Read the model definition and answer for the solid it produces. Units are mm, in the model's axes. Face numbers are marked on the shaded views. A direction names the side the tool comes from. Round coordinates to 2 decimals unless told otherwise and drop trailing zeros. Order: outer loops, then holes, each group sorted by start corner. A loop starts at its lowest first (then second) coordinate and runs counter-clockwise, first axis right, second up. Notation, with made-up numbers: (40.25, 29) - (64.25, 29) arc R27 cw to (64.25, 60) - close; hole circle Ø10 at (50, -19.75). An arc over 180 degrees is marked (long way). Put each result on its own line as item: value. Start each with the question number.
Q1. Which of the six approach directions +Z, -Z, +X, -X, +Y, -Y give full straight-line access (tool end or side, diameter ignored) to the marked faces 4 and 5?
Q2. Find the intervals of material crossed by line 1 along X through (y, z) = (10.5, 21); line 2 along Y through (x, z) = (29, 48.5); line 3 along X through (y, z) = (22.5, 43), in increasing order. Write a range as from..to.
Q3. For a pull along X with two mould halves and no side action, classify the marked faces 1, 2 and 3 as pulls with the +X half, pulls with the -X half, needs draft (parallel to the pull), parting line crosses it, or undercut.
Q4. Section C-C on y = 7.75 is taken. Give the vertices of the cut face in (x, z).
Q5. Section B-B on z = 31 is taken. Give the vertices of the cut face in (x, y).
Q6. Section D-D on x = 9.5 is taken. Give the vertices of the cut face in (y, z).
Q7. Each of these flat-tipped pins is pushed along its axis until it touches: pin 1 Ø8 at (x, y) = (16.5, 20.5) entering from +Z; pin 2 Ø22.5 at (x, z) = (25, 67.5) entering from +Y; pin 3 Ø2.5 at (x, y) = (7.5, 18.5) entering from -Z. Where does it stop, or does it pass through?
Q8. Section A-A on y = 21.5 is taken. Give the vertices of the cut face in (x, z), then the cut area to 3 significant figures.
Autodesk Inventor part; units mm, degrees
ref_plane "YZ Plane" through (0, 0, 0) normal (1, 0, 0) x (0, 1, 0)
ref_plane "XZ Plane" through (0, 0, 0) normal (0, 1, 0) x (-1, 0, 0)
ref_plane "XY Plane" through (0, 0, 0) normal (0, 0, 1) x (1, 0, 0)
sketch "Sketch1" plane through (0, 0, 0) normal (0, 0, 1) x (1, 0, 0)
  line L0 (10.7104, 9.7791) -> (45.7104, 9.7791)
  line L1 (45.7104, 9.7791) -> (45.7104, 24.7791)
  line L2 (10.7104, 9.7791) -> (10.7104, 24.7791)
  line L3 (5.7104, 24.7791) -> (5.7104, 4.7791)
  line L4 (5.7104, 4.7791) -> (50.7104, 4.7791)
  line L5 (50.7104, 4.7791) -> (50.7104, 24.7791)
  line L6 (5.7104, 24.7791) -> (10.7104, 24.7791)
  line L7 (45.7104, 24.7791) -> (50.7104, 24.7791)
  point P0 (0, 0)
  point P1 (28.2104, 9.7791)
  dimension "d0" = 35
  dimension "d1" = 15
  dimension "d2" = 15
  dimension "d29" = 5
extrude "Extrusion1" add sketch "Sketch1" along normal blind 100
sketch "Sketch3" plane through (10.7104, 9.7791, 0) normal (0, 1, 0) x (1, 0, 0)
  line L0 (-5, -100) -> (40, -100)
  line L1 (-5, 0) -> (-5, -100)
  line L2 (17.5, -100) -> (37.1919, -100) construction
  line L3 (-5, -85.7353) -> (-5, -100)
  line L4 (-5, -100) -> (17.5, -100)
  line L5 (40, 0) -> (40, -100)
  line L6 (17.5, -100) -> (37.1919, -100) construction
  line L7 (40, -85.7353) -> (40, -100)
  line L8 (40, -100) -> (17.5, -100)
  line L9 (40, 0) -> (40, -100)
  line L10 (17.5, -100) -> (-5, -36.462)
  line L11 (17.5, -100) -> (40, -36.462)
  line L12 (-5, -36.462) -> (40, -36.462)
  line L13 (35, 0) -> (35, -100)
  line L14 (0, 0) -> (0, -100)
  point P0 (-10.7104, 0)
  point P1 (-5, -77.7514)
  point P2 (40, -36.462)
  point P3 (-5, -60.8533)
  dimension "d33" = 39
extrude "Extrusion5" cut sketch "Sketch3" along normal through all both and the other way through all contours L1 L10 L14 L0 | L14 L10 L0 | L11 L13 L0 | L13 L11 L5 L0
sketch "Sketch4" plane through (50.7104, 4.7791, 0) normal (1, 0, 0) x (0, 0, -1)
  line L0 (0, 20) -> (-50.5815, 20)
  line L1 (0, 20) -> (-4, 20)
  line L2 (-4, 20) -> (-4, 5)
  line L3 (0, 5) -> (-50.5815, 5)
  line L4 (0, 20) -> (0, 5)
  line L5 (0, 5) -> (0, 20)
  line L6 (0, 20) -> (0, 5)
  line L7 (-4, 5) -> (0, 5)
  point P0 (0, -4.7791)
  dimension "d24" = 4
extrude "Extrusion6" cut sketch "Sketch4" against normal through all
equation "\"BendRadius\" = Thickness"
equation "\"BendReliefWidth\" = Thickness"
equation "\"BendReliefDepth\" = 0.5 * Thickness"
equation "\"CornerReliefSize\" = 4 * Thickness"
equation "\"MinimumRemnant\" = 2 * Thickness"
equation "\"TransitionRadius\" = BendRadius"
equation "\"JacobiRadiusSize\" = BendRadius"
equation "\"GapSize\" = Thickness"
properties part number "middleslide2"
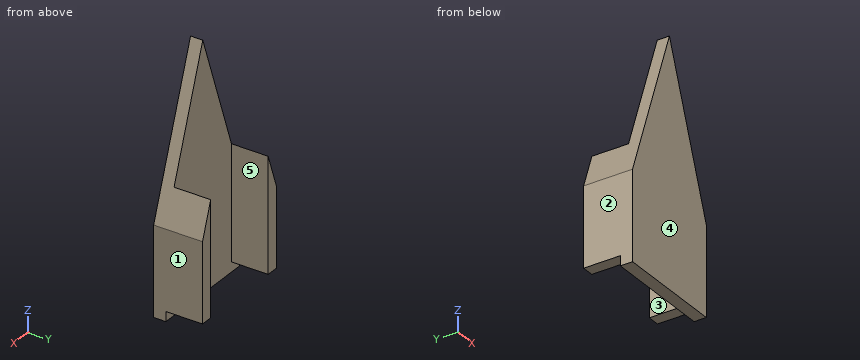
Findings:
1. face 4: +Z, -Z, +X, -X, -Y
1. face 5: +Z, -Z, +Y
2. line 1: 5.71..10.71, 45.71..50.71
2. line 2: 4.78..9.78
2. line 3: 8.03..10.71, 45.71..48.4
3. face 1: pulls with the +X half
3. face 2: pulls with the -X half
3. face 3: undercut
4. outline: (5.71, 0) - (50.71, 0) - (50.71, 36.46) - (28.21, 100) - (5.71, 36.46) - close
5. outline: (5.71, 4.78) - (50.71, 4.78) - (50.71, 24.78) - (45.71, 24.78) - (45.71, 9.78) - (10.71, 9.78) - (10.71, 24.78) - (5.71, 24.78) - close
6. outline: (4.78, 0) - (9.78, 0) - (9.78, 4) - (24.78, 4) - (24.78, 47.16) - (4.78, 47.16) - close
7. pin 1: through
7. pin 2: y = 9.78
7. pin 3: z = 4
8. outline: (5.71, 4) - (10.71, 4) - (10.71, 50.58) - (5.71, 36.46) - close; (45.71, 4) - (50.71, 4) - (50.71, 36.46) - (45.71, 50.58) - close
8. area: 395 mm2
